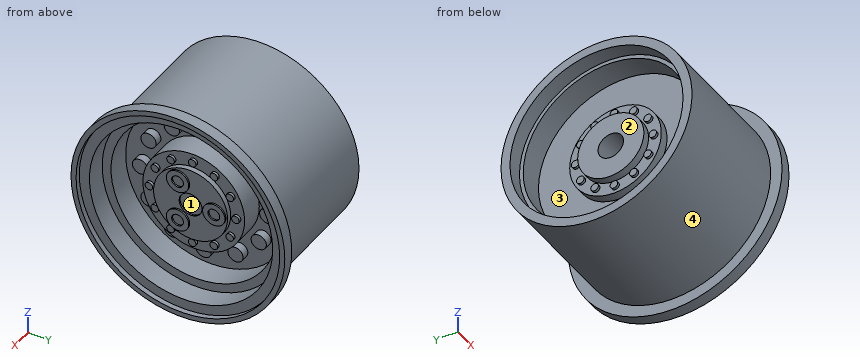
```python
from build123d import *

# Parameters (mm, degrees)
SKETCH2_R           = 0.75
BOSS_EXTRUDE1_DEPTH = 0.75
SKETCH3_R           = 0.375
BOSS_EXTRUDE2_DEPTH = 0.25
SKETCH5_R           = 1.125
CUT_EXTRUDE1_DEPTH  = 0.15
SKETCH6_R           = 1.1
SKETCH6_R_2         = 0.575
BOSS_EXTRUDE3_DEPTH = 0.15
SKETCH7_R           = 0.375
BOSS_EXTRUDE4_DEPTH = 0.25
SKETCH8_R           = 1.25
CUT_EXTRUDE2_DEPTH  = 5


with BuildPart() as part:
    # Sketch1 → Revolve1 (revolve)
    with BuildSketch(Plane.XY):
        Polygon((3.75, 0), (0, 0), (-5.5, 0), (-5.5, 3.25), (-4.75, 3.25), (-4.75, 4.5), (-3.85, 4.5), (-3.85, 8.13), (-6.25, 8.13), (-6.25, 8.5), (-7.75, 8.5), (-7.75, 9.38), (0, 9.38), (4.65, 9.38), (4.65, 10.5), (5.75, 10.5), (5.75, 10), (5.25, 10), (5.25, 9), (3.25, 9), (3.25, 8.13), (0.943, 8.13), (0.943, 5), (3.25, 5), (3.25, 3.63), (3.75, 3.63), align=None)
    revolve(axis=Axis((0, 0, 0), (-1, 0, 0)))

    # Sketch2 → Boss-Extrude1 (add)
    with BuildSketch(Plane(origin=(0.943, 0, 0), x_dir=(0, 0, -1), z_dir=(1, 0, 0))):
        with Locations(Location((0, 6.25, 0), (0, 0, 90))):
            Circle(SKETCH2_R)
        with Locations(Location((3.125, 5.412658774, 0), (0, 0, 90))):
            Circle(SKETCH2_R)
        with Locations(Location((5.412658774, 3.125, 0), (0, 0, 90))):
            Circle(SKETCH2_R)
        with Locations(Location((6.25, 0, 0), (0, 0, 90))):
            Circle(SKETCH2_R)
        with Locations(Location((5.412658774, -3.125, 0), (0, 0, 90))):
            Circle(SKETCH2_R)
        with Locations(Location((3.125, -5.412658774, 0), (0, 0, 90))):
            Circle(SKETCH2_R)
        with Locations(Location((0, -6.25, 0), (0, 0, 90))):
            Circle(SKETCH2_R)
        with Locations(Location((-3.125, -5.412658774, 0), (0, 0, 90))):
            Circle(SKETCH2_R)
        with Locations(Location((-5.412658774, -3.125, 0), (0, 0, 90))):
            Circle(SKETCH2_R)
        with Locations(Location((-6.25, 0, 0), (0, 0, 90))):
            Circle(SKETCH2_R)
        with Locations(Location((-5.412658774, 3.125, 0), (0, 0, 90))):
            Circle(SKETCH2_R)
        with Locations(Location((-3.125, 5.412658774, 0), (0, 0, 90))):
            Circle(SKETCH2_R)
    extrude(amount=BOSS_EXTRUDE1_DEPTH)

    # Sketch3 → Boss-Extrude2 (add)
    with BuildSketch(Plane(origin=(3.25, 0, 0), x_dir=(0, 0, -1), z_dir=(1, 0, 0))):
        with Locations(Location((0, 4.25, 0), (0, 0, 90))):
            Circle(SKETCH3_R)
        with Locations(Location((2.125, 3.680607966, 0), (0, 0, 90))):
            Circle(SKETCH3_R)
        with Locations(Location((3.680607966, 2.125, 0), (0, 0, 90))):
            Circle(SKETCH3_R)
        with Locations(Location((4.25, 0, 0), (0, 0, 90))):
            Circle(SKETCH3_R)
        with Locations(Location((3.680607966, -2.125, 0), (0, 0, 90))):
            Circle(SKETCH3_R)
        with Locations(Location((2.125, -3.680607966, 0), (0, 0, 90))):
            Circle(SKETCH3_R)
        with Locations(Location((0, -4.25, 0), (0, 0, 90))):
            Circle(SKETCH3_R)
        with Locations(Location((-2.125, -3.680607966, 0), (0, 0, 90))):
            Circle(SKETCH3_R)
        with Locations(Location((-3.680607966, -2.125, 0), (0, 0, 90))):
            Circle(SKETCH3_R)
        with Locations(Location((-4.25, 0, 0), (0, 0, 90))):
            Circle(SKETCH3_R)
        with Locations(Location((-3.680607966, 2.125, 0), (0, 0, 90))):
            Circle(SKETCH3_R)
        with Locations(Location((-2.125, 3.680607966, 0), (0, 0, 90))):
            Circle(SKETCH3_R)
    extrude(amount=BOSS_EXTRUDE2_DEPTH)

    # Sketch5 → Cut-Extrude1 (cut)
    with BuildSketch(Plane(origin=(3.75, 0, 0), x_dir=(0, 0, -1), z_dir=(1, 0, 0))):
        with Locations(Location((0, 0, 0), (0, 0, 90))):
            Circle(SKETCH5_R)
    extrude(amount=-CUT_EXTRUDE1_DEPTH, mode=Mode.SUBTRACT)

    # Sketch6 → Boss-Extrude3 (add)
    # profile 1 of 3: a face of its own
    with BuildSketch(Plane(origin=(3.75, 0, 0), x_dir=(0, 0, -1), z_dir=(1, 0, 0))):
        with Locations(Location((0, 2.375, 0), (0, 0, 90))):
            Circle(SKETCH6_R)
        with Locations(Location((0, 2.375, 0), (0, 0, 90))):
            Circle(SKETCH6_R_2, mode=Mode.SUBTRACT)
    # profile 2 of 3: a face of its own
    with BuildSketch(Plane(origin=(3.75, 0, 0), x_dir=(0, 0, -1), z_dir=(1, 0, 0))):
        with Locations(Location((2.056810334, -1.1875, 0), (0, 0, 90))):
            Circle(SKETCH6_R)
        with Locations(Location((2.056810334, -1.1875, 0), (0, 0, 90))):
            Circle(SKETCH6_R_2, mode=Mode.SUBTRACT)
    # profile 3 of 3: a face of its own
    with BuildSketch(Plane(origin=(3.75, 0, 0), x_dir=(0, 0, -1), z_dir=(1, 0, 0))):
        with Locations(Location((-2.056810334, -1.1875, 0), (0, 0, 90))):
            Circle(SKETCH6_R)
        with Locations(Location((-2.056810334, -1.1875, 0), (0, 0, 90))):
            Circle(SKETCH6_R_2, mode=Mode.SUBTRACT)
    extrude(amount=BOSS_EXTRUDE3_DEPTH)

    # Sketch7 → Boss-Extrude4 (add)
    with BuildSketch(Plane.ZY.offset(4.75)):
        with Locations(Location((0, 3.81, 0), (0, 0, 270))):
            Circle(SKETCH7_R)
        with Locations(Location((1.905, 3.299556788, 0), (0, 0, 270))):
            Circle(SKETCH7_R)
        with Locations(Location((3.299556788, 1.905, 0), (0, 0, 270))):
            Circle(SKETCH7_R)
        with Locations(Location((3.81, 0, 0), (0, 0, 270))):
            Circle(SKETCH7_R)
        with Locations(Location((3.299556788, -1.905, 0), (0, 0, 270))):
            Circle(SKETCH7_R)
        with Locations(Location((1.905, -3.299556788, 0), (0, 0, 270))):
            Circle(SKETCH7_R)
        with Locations(Location((0, -3.81, 0), (0, 0, 270))):
            Circle(SKETCH7_R)
        with Locations(Location((-1.905, -3.299556788, 0), (0, 0, 270))):
            Circle(SKETCH7_R)
        with Locations(Location((-3.299556788, -1.905, 0), (0, 0, 270))):
            Circle(SKETCH7_R)
        with Locations(Location((-3.81, 0, 0), (0, 0, 270))):
            Circle(SKETCH7_R)
        with Locations(Location((-3.299556788, 1.905, 0), (0, 0, 270))):
            Circle(SKETCH7_R)
        with Locations(Location((-1.905, 3.299556788, 0), (0, 0, 270))):
            Circle(SKETCH7_R)
    extrude(amount=BOSS_EXTRUDE4_DEPTH)

    # Sketch8 → Cut-Extrude2 (cut)
    with BuildSketch(Plane.ZY.offset(5.5)):
        with Locations(Location((0, 0, 0), (0, 0, 270))):
            Circle(SKETCH8_R)
    extrude(amount=-CUT_EXTRUDE2_DEPTH, mode=Mode.SUBTRACT)


solid = part.part
```
Input: part model. Units: mm. Frame: model coordinates. Face numbers are marked on the shaded views. A direction names the side the tool comes from. Give positions to 0.01 mm unless a question says otherwise; leave off trailing zeros. Write each loop counter-clockwise with the first axis right and the second up, starting at its lowest first coordinate (ties: lowest second). Pieces come first, ordered by that corner, then holes. Notation, with made-up numbers: (31, 27) - (49, 27) arc R18 ccw to (49, 52) - close; hole circle Ø4 at (32, -21.5). An arc over 180 degrees is marked (long way). Write item = value, one per line. Start each with the question number.
1. Access query for the marked faces 1 and 2. Directions: +Z, -Z, +X, -X, +Y, -Y. A direction counts if a zero-diameter tool reaches every point of the face in a straight line with its end or side. Return the directions, or none.
2. Section query B-B, the plane x = -1. Output: boundary loops of the cut face in (y, z), then the cut area to 3 significant figures.
3. Mould query, pull axis Y, two halves, no side actions, for the marked faces 3 and 4. Classes: released by +Y, released by -Y, zero draft, split by the parting line, or undercut.
4. First-contact query: pin 1 Ø1 at (x, y) = (0.5, 4) entering from +Z; pin 2 Ø2 at (y, z) = (0, 0) entering from +X; pin 3 Ø0.8 at (y, z) = (-2.5, -3.5) entering from +X. Flat tips, straight axial feed; report the tip coordinate or a pass-through.
5. Ray query, L1, parallel to Z at x = -5.15, y = 0; L2, parallel to Z at x = -4.2, y = 0; L3, parallel to Y at x = 2.25, z = 0. Return the intervals inside material, ascending.
6. Section query A-A, the plane y = -7.5. Output: boundary loops of the cut face in (x, z), then the cut area to 3 significant figures.
Check sheet entries:
q1.face_1 = +X
q1.face_2 = -X
q2.outline = circle Ø18.76 at (0, 0); hole circle Ø2.5 at (0, 0)
q2.area = 272 mm2
q3.face_3 = undercut
q3.face_4 = split by the parting line
q4.pin_1 = 8.7
q4.pin_2 = 3.6
q4.pin_3 = 3.5
q5.L1 = -9.38 to -8.13, -3.25 to -1.25, 1.25 to 3.25, 8.13 to 9.38
q5.L2 = -9.38 to -8.13, -4.5 to -1.25, 1.25 to 4.5, 8.13 to 9.38
q5.L3 = -9.38 to -8.13, -5 to 5, 8.13 to 9.38
q6.outline = (-7.75, -5.63) - (4.65, -5.63) - (4.65, -7.35) - (5.75, -7.35) - (5.75, -6.61) - (5.25, -6.61) - (5.25, -4.97) - (3.25, -4.97) - (3.25, -3.14) - (0.94, -3.14) - (0.94, 3.14) - (3.25, 3.14) - (3.25, 4.97) - (5.25, 4.97) - (5.25, 6.61) - (5.75, 6.61) - (5.75, 7.35) - (4.65, 7.35) - (4.65, 5.63) - (-7.75, 5.63) - (-7.75, 4) - (-6.25, 4) - (-6.25, 3.14) - (-3.85, 3.14) - (-3.85, -3.14) - (-6.25, -3.14) - (-6.25, -4) - (-7.75, -4) - close
q6.area = 87.8 mm2
